from build123d import *

# Parameters (mm, degrees)
SKETCH1_W           = 30
SKETCH1_H           = 24
BOSS_EXTRUDE1_DEPTH = 1
SKETCH3_R           = 2
CUT_EXTRUDE1_DEPTH  = 3
CHAMFER1_SIZE       = 8


with BuildPart() as part:
    # Sketch1 → Boss-Extrude1 (new body)
    with BuildSketch(Plane.XY):
        Rectangle(SKETCH1_W, SKETCH1_H)
    extrude(amount=BOSS_EXTRUDE1_DEPTH)

    # Sketch3 → Cut-Extrude1 (cut)
    with BuildSketch(Plane(origin=(0, 0, 0), x_dir=(-1, 0, 0), z_dir=(0, 0, -1))):
        with Locations((-4.5, 6)):
            Circle(SKETCH3_R)
        with Locations((-4.5, -6)):
            Circle(SKETCH3_R)
        with Locations((-10.5, 0)):
            Circle(SKETCH3_R)
    cut_extrude1 = extrude(amount=-CUT_EXTRUDE1_DEPTH, mode=Mode.SUBTRACT)

    # Chamfer1
    chamfer1_edges = [part.edges().sort_by_distance(p)[0] for p in [
        (15, -12, 0.5),
        (15, 12, 0.5),
        (-15, 12, 0.5),
        (-15, -12, 0.5),
    ]]
    chamfer(chamfer1_edges, length=CHAMFER1_SIZE)

    # Mirror1: Cut-Extrude1 across plane
    add(cut_extrude1.mirror(Plane(origin=(0, 0, 0), x_dir=(0, 0, 1), z_dir=(1, 0, 0))), mode=Mode.SUBTRACT)


solid = part.part
Geometry: final body of the model. Coordinates: model frame, mm. Coordinates: 2 decimals unless noted, no trailing zeros. Loops run counter-clockwise (first coordinate to the right, second up) from the corner with the lowest first, then second, coordinate; pieces in that order, holes last. Notation, with made-up numbers: M 75.5,69.5 L 119.5,69.5 A27 cw 119.5,91.5 Z; hole C 86,11.25 d5. An arc over 180 degrees is marked long. One line per item, written item: value. Start each with the question number.
1) Cut plane B-B (x = -10.5). Return loops of the section in (y, z), then the cut area to 3 significant figures.
2) Material intervals for L1, parallel to Y at x = 4.5, z = 0.4; L2, parallel to Y at x = 6, z = 0.6; L3, parallel to X at y = -1.5, z = 0.4, sorted ascending. Write a range as from..to.
3) Cut plane C-C (z = 0.8). Return loops of the section in (x, y).
4) Cut plane A-A (y = 6). Return loops of the section in (x, z).
5) Cut plane D-D (x = 4.5). Return loops of the section in (y, z).
6) Pin query (flat end, axial travel): P1, Ø3, axis at x = 10.5, y = 0, coming from the +Z side (3 decimals); P2, Ø5, axis at x = 4.5, y = 6, coming from the -Z side. Return the tip coordinate at first contact, or that it passes through.
7) Draft query along Y for faces 1 (the cylindrical face through (5.974, 7.352, 0.493)), 2 (the flat face through (-0.1, -12, 0.5)), 3 (the flat face through (0, 0, 1)). Return one class per face: released by +Y, released by -Y, zero draft, split by the parting line, or undercut.
Evaluation:
1. outline: M -8.5,0 L -2,0 L -2,1 L -8.5,1 Z; M 2,0 L 8.5,0 L 8.5,1 L 2,1 Z
1. area: 13.0 mm^2
2. L1: -12..-8, -4..4, 8..12
2. L2: -12..-7.32, -4.68..4.68, 7.32..12
2. L3: -15..-11.82, -9.18..9.18, 11.82..15
3. outline: M -15,-4 L -7,-12 L 7,-12 L 15,-4 L 15,4 L 7,12 L -7,12 L -15,4 Z; hole C -10.5,0 d4; hole C -4.5,-6 d4; hole C -4.5,6 d4; hole C 4.5,-6 d4; hole C 4.5,6 d4; hole C 10.5,0 d4
4. outline: M -13,0 L -6.5,0 L -6.5,1 L -13,1 Z; M -2.5,0 L 2.5,0 L 2.5,1 L -2.5,1 Z; M 6.5,0 L 13,0 L 13,1 L 6.5,1 Z
5. outline: M -12,0 L -8,0 L -8,1 L -12,1 Z; M -4,0 L 4,0 L 4,1 L -4,1 Z; M 8,0 L 12,0 L 12,1 L 8,1 Z
6. P1: through
6. P2: z = 0
7. face 1: undercut
7. face 2: released by -Y
7. face 3: zero draft
